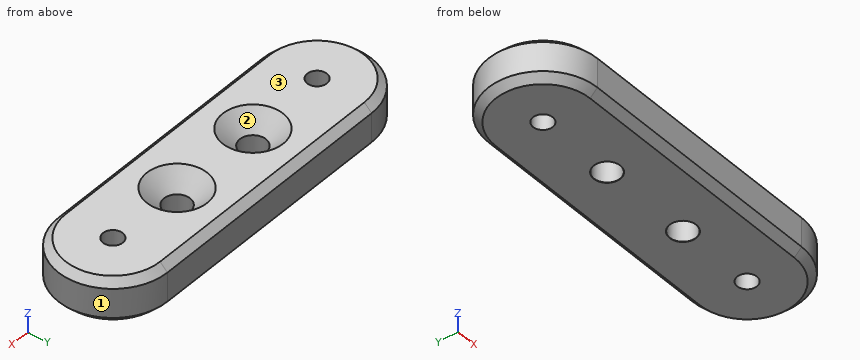
```python
from build123d import *

# Parameters (mm, degrees)
SKETCH1_R                                    = 1.35
BOSS_EXTRUDE1_DEPTH                          = 6
CHAMFER1_SIZE                                = 1
CSK_FOR_M3_COUNTERSUNK_FLAT_HEAD_SCR_2_COUNT = 2
CSK_FOR_M3_COUNTERSUNK_FLAT_HEAD_SCR_2_PITCH = 13


with BuildPart() as part:
    # Sketch1 → Boss-Extrude1 (new body)
    with BuildSketch(Plane.XY):
        with BuildLine():
            Line((-17.5, 7.5), (17.5, 7.5))
            ThreePointArc((17.5, 7.5), (25, 0), (17.5, -7.5))
            Line((17.5, -7.5), (-17.5, -7.5))
            ThreePointArc((-17.5, -7.5), (-25, 0), (-17.5, 7.5))
        make_face()
        with Locations((-17.5, 0)):
            Circle(SKETCH1_R, mode=Mode.SUBTRACT)
        with Locations((17.5, 0)):
            Circle(SKETCH1_R, mode=Mode.SUBTRACT)
    extrude(amount=BOSS_EXTRUDE1_DEPTH)

    # Chamfer1
    chamfer1_edges = [part.edges().sort_by_distance(p)[0] for p in [
        (25, 0, 6),
        (0, 7.5, 6),
        (-25, 0, 6),
        (0, 7.5, 0),
        (25, 0, 0),
        (0, -7.5, 0),
        (-25, 0, 0),
        (0, -7.5, 6),
    ]]
    chamfer(chamfer1_edges, length=CHAMFER1_SIZE)

    # Sketch3 → CSK for M3 Countersunk Flat Head Screw1 (revolve, cut)
    with BuildSketch(Plane(origin=(6.5, 0, 6), x_dir=(0, -1, 0), z_dir=(1, 0, 0))):
        Polygon((0, 0), (0, 6), (1.825, 6), (1.8, 5.975), (1.8, 2.35), (4.15, 0), align=None)
    csk_for_m3_countersunk_flat_head_screw1 = revolve(axis=Axis((6.5, 0, 12.35), (0, 0, -1)), mode=Mode.SUBTRACT)

    # CSK for M3 Countersunk Flat Head Scr 2: CSK for M3 Countersunk Flat Head Screw1 ×2
    with Locations(*[(-i * CSK_FOR_M3_COUNTERSUNK_FLAT_HEAD_SCR_2_PITCH, 0, 0) for i in range(1, CSK_FOR_M3_COUNTERSUNK_FLAT_HEAD_SCR_2_COUNT)]):
        add(csk_for_m3_countersunk_flat_head_screw1, mode=Mode.SUBTRACT)


solid = part.part
```
Could you check a few things on this model? Use its own coordinates, in mm. Face numbers are marked on the shaded views. Give positions to 0.01 mm unless a question says otherwise; leave off trailing zeros. Order: outer loops, then holes, each group sorted by start corner. A loop starts at its lowest first (then second) coordinate and runs counter-clockwise, first axis right, second up.
Q1. Suppose I cut it at C-C, the plane y = 0. Count the separate pieces of the cut face and the enclosed holes in it, and give its area (3 significant figures).
Q2. Suppose I cut it at B-B, the plane z = 0.5. Write out the boundary of the cut face in (x, y), and give its area (3 significant figures).
Q3. We'd pull the mould along Y, two halves only. Please class the marked faces 1, 2 and 3: +Y half, -Y half, draft (parallel to the pull), parting line (faces both ways), or undercut.
Q4. I'm going to push flat-ended pins straight in: P1, Ø2, axis at x = 6.5, y = 0, coming from the +Z side; P2, Ø3, axis at y = -3, z = 1, coming from the -X side; P3, Ø4, axis at x = -6.5, y = 0, coming from the +Z side; P4, Ø1.5, axis at x = 8, y = 0, coming from the +Z side. Where does each tip first touch, or does it pass through?
Q5. If I drill on line 1 along Y through (x, z) = (-17.5, 1.6); line 2 along X through (y, z) = (1, 4.4); line 3 along Y through (x, z) = (7, 3.6), over which ranges is the centre line in solid material (lowest first)?
Q6. Suppose I cut it at D-D, the plane z = 4.55. Write out the boundary of the cut face in (x, y).
Q7. Suppose I cut it at A-A, the plane x = 6.5. Write out the boundary of the cut face in (y, z) (3 decimals).
Solution:
1. separate pieces: 5
1. enclosed holes: 0
1. area: 211 mm2
2. outline: (-17.5, -7) - (17.5, -7) arc R7 ccw to (17.5, 7) - (-17.5, 7) arc R7 ccw to start; hole circle Ø2.7 at (-17.5, 0); hole circle Ø3.6 at (-6.5, 0); hole circle Ø3.6 at (6.5, 0); hole circle Ø2.7 at (17.5, 0)
2. area: 612 mm2
3. face 1: parting line
3. face 2: undercut
3. face 3: draft
4. P1: passes through
4. P2: stops at x = -24.85
4. P3: stops at z = 3.85
4. P4: stops at z = 4.1
5. line 1: y = -7.5 to -1.35, 1.35 to 7.5
5. line 2: x = -24.93 to -18.41, -16.59 to -8.85, -4.15 to 4.15, 8.85 to 16.59, 18.41 to 24.93
5. line 3: y = -7.5 to -1.73, 1.73 to 7.5
6. outline: (-17.5, -7.5) - (17.5, -7.5) arc R7.5 ccw to (17.5, 7.5) - (-17.5, 7.5) arc R7.5 ccw to start; hole circle Ø2.7 at (-17.5, 0); hole circle Ø5.4 at (-6.5, 0); hole circle Ø5.4 at (6.5, 0); hole circle Ø2.7 at (17.5, 0)
7. outline: (-7.5, 1) - (-6.5, 0) - (-1.825, 0) - (-1.8, 0.025) - (-1.8, 3.65) - (-4.15, 6) - (-6.5, 6) - (-7.5, 5) - close; (1.8, 0.025) - (1.825, 0) - (6.5, 0) - (7.5, 1) - (7.5, 5) - (6.5, 6) - (4.15, 6) - (1.8, 3.65) - close
